For this review, use the dimensioned drawing (mm, ordinates from the lowest corner) and the shaded views. A direction names the side the tool comes from. Coordinates: 2 decimals unless noted, no trailing zeros. Write each loop counter-clockwise with the first axis right and the second up, starting at its lowest first coordinate (ties: lowest second). Pieces come first, ordered by that corner, then holes. Notation, with made-up numbers: (47.5, -21) - (76.5, -21) arc R10 cw to (76.5, -10) - close; hole circle Ø9 at (18, 12). An arc over 180 degrees is marked (long way). One line per item, written item: value.
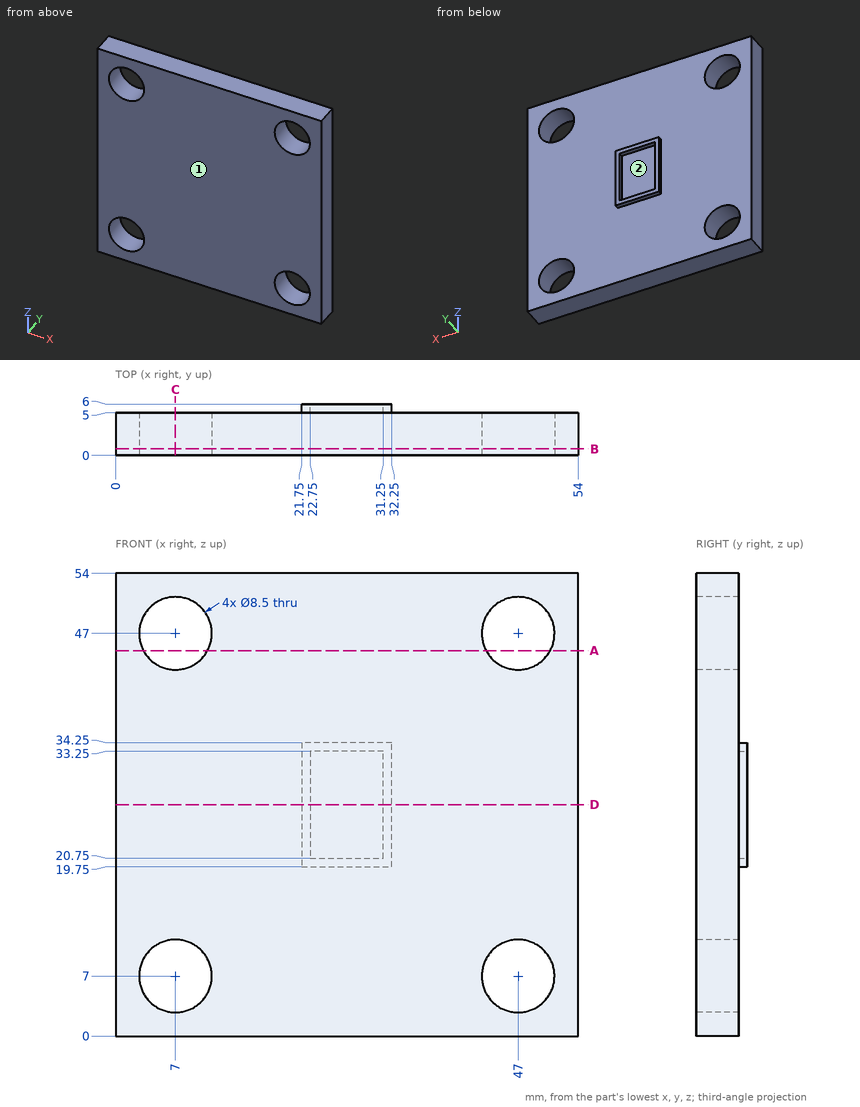
1. For the marked faces 1 and 2, list the 3-axis set-ups (+Z, -Z, +X, -X, +Y, -Y) from which the entire face can be reached by the end or side of a thin tool; tool diameter is ignored.
Answer block:
face 1: +Z, -Z, +X, -X, -Y
face 2: +Y
2. Consider section B-B, the plane y = 0.75. Write out the cut boundary in (x, z), then the cut area to 3 significant figures.
Answer block:
outline: (0, 0) - (54, 0) - (54, 54) - (0, 54) - close; hole circle Ø8.5 at (7, 7); hole circle Ø8.5 at (7, 47); hole circle Ø8.5 at (47, 7); hole circle Ø8.5 at (47, 47)
area: 2,690 mm^2
3. Insertion check: pin 1 Ø10 at (x, z) = (47, 7) entering from +Y; pin 2 Ø0.5 at (y, z) = (5.5, 28) entering from -X; pin 3 Ø0.8 at (x, y) = (25.5, 5.5) entering from -Z. Each pin has a flat end and moves straight along its axis. Give the tip position at first contact, or say it passes through.
Answer block:
pin 1: stops at y = 5
pin 2: stops at x = 21.75
pin 3: stops at z = 19.75
4. Consider section A-A, the plane z = 45. Write out the cut boundary in (x, y), then the cut area to 3 significant figures.
Answer block:
outline: (0, 0) - (3.25, 0) - (3.25, 5) - (0, 5) - close; (10.75, 0) - (43.25, 0) - (43.25, 5) - (10.75, 5) - close; (50.75, 0) - (54, 0) - (54, 5) - (50.75, 5) - close
area: 195 mm^2
5. Consider section D-D, the plane z = 27. Write out the cut boundary in (x, y), then the cut area to 3 significant figures.
Answer block:
outline: (0, 0) - (54, 0) - (54, 5) - (32.25, 5) - (32.25, 6) - (31.25, 6) - (31.25, 5) - (22.75, 5) - (22.75, 6) - (21.75, 6) - (21.75, 5) - (0, 5) - close
area: 272 mm^2
6. Wall thickness on line 1 along X through (y, z) = (2.5, 7); line 2 along X through (y, z) = (1.65, 8.5): over which ranges is each line inside the solid? List them lowest first.
Answer block:
line 1: x = 0 to 2.75, 11.25 to 42.75, 51.25 to 54
line 2: x = 0 to 3.02, 10.98 to 43.02, 50.98 to 54
7. Consider section C-C, the plane x = 7. Write out the cut boundary in (y, z).
Answer block:
outline: (0, 0) - (5, 0) - (5, 2.75) - (0, 2.75) - close; (0, 11.25) - (5, 11.25) - (5, 42.75) - (0, 42.75) - close; (0, 51.25) - (5, 51.25) - (5, 54) - (0, 54) - close
